The model under review builds one solid part; all positions refer to its coordinate system, in mm. A direction names the side the tool comes from. Give positions to 0.01 mm unless a question says otherwise; leave off trailing zeros. Order: outer loops, then holes, each group sorted by start corner. A loop starts at its lowest first (then second) coordinate and runs counter-clockwise, first axis right, second up.
Autodesk Inventor part; units mm, degrees
ref_plane "YZ Plane" through (0, 0, 0) normal (1, 0, 0) x (0, 1, 0)
ref_plane "XZ Plane" through (0, 0, 0) normal (0, 1, 0) x (-1, 0, 0)
ref_plane "XY Plane" through (0, 0, 0) normal (0, 0, 1) x (1, 0, 0)
sketch "Sketch1" plane through (0, 0, 0) normal (0, 1, 0) x (-1, 0, 0)
  point P0 (0, 0)
sketch "Sketch2" plane through (0, 0, 0) normal (0, 1, 0) x (-1, 0, 0)
  arc A0 (0, -12.775) -> (0, 12.775) centre (0, 0) ccw
  arc A1 (0, -27.775) -> (0, 27.775) centre (0, 0) ccw
  line L0 (0, 27.775) -> (0, -27.775)
  dimension "d0" = 25.55
  dimension "d1" = 15
extrude "Extrusion1" add sketch "Sketch2" along normal blind 14 contours A0 L0 A1
sketch "Sketch4" plane through (0, 0, 27.775) normal (1, 0, 0) x (0, 0, -1)
  line L0 (4.7364, 11.7377) -> (10.2211, 11.7622)
  line L1 (10.2211, 11.7622) -> (12.9848, 7.0245)
  line L2 (12.9848, 7.0245) -> (10.2636, 2.2623)
  line L3 (10.2636, 2.2623) -> (4.7789, 2.2378)
  line L4 (4.7789, 2.2378) -> (2.0152, 6.9755)
  line L5 (2.0152, 6.9755) -> (4.7364, 11.7377)
  line L6 (0, 14) -> (15, 14)
  line L7 (0, 0) -> (0, 14)
  line L8 (15, 14) -> (40.55, 14)
  line L9 (27.775, 14) -> (27.775, 0)
  line L10 (50.8136, 11.7377) -> (45.3289, 11.7622)
  line L11 (45.3289, 11.7622) -> (42.5652, 7.0245)
  line L12 (42.5652, 7.0245) -> (45.2864, 2.2623)
  line L13 (45.2864, 2.2623) -> (50.7711, 2.2378)
  line L14 (50.7711, 2.2378) -> (53.5348, 6.9755)
  line L15 (53.5348, 6.9755) -> (50.8136, 11.7377)
  line L16 (55.55, 14) -> (40.55, 14)
  line L17 (55.55, 0) -> (55.55, 14)
  line L18 (40.55, 14) -> (15, 14)
  point P0 (7.5, 7)
  point P1 (7.4787, 11.75)
  point P2 (7.5, 14)
  point P3 (0, 7)
  point P4 (48.05, 7)
  point P5 (48.0713, 11.75)
  point P6 (48.05, 14)
  point P7 (55.55, 7)
  dimension "d5" = 9.5
  dimension "d6" = 0
  dimension "d7" = 0
extrude "Extrusion2" cut sketch "Sketch4" against normal through all
sketch "Sketch5" plane through (0, 0, 27.775) normal (1, 0, 0) x (0, 0, -1)
  line L0 (4.7364, 11.7377) -> (10.2211, 11.7622)
  circle A0 centre (7.4787, 6.9999) radius 2.85
  line L1 (0.8522, 11.9261) -> (14.3606, 11.9261)
  line L2 (14.3606, 11.9261) -> (14.3606, 2.2036)
  line L3 (14.3606, 2.2036) -> (0.8522, 2.2036)
  line L4 (0.8522, 2.2036) -> (0.8522, 11.9261)
  line L5 (10.2636, 2.2623) -> (4.7789, 2.2378)
  line L6 (55.55, 14) -> (0, 14)
  line L7 (27.775, 14) -> (27.775, 0)
  line L8 (55.55, 0) -> (0, 0)
  line L9 (50.8136, 11.7377) -> (45.3289, 11.7622)
  circle A1 centre (48.0713, 6.9999) radius 2.85
  line L10 (54.6978, 11.9261) -> (41.1894, 11.9261)
  line L11 (41.1894, 11.9261) -> (41.1894, 2.2036)
  line L12 (41.1894, 2.2036) -> (54.6978, 2.2036)
  line L13 (54.6978, 2.2036) -> (54.6978, 11.9261)
  line L14 (45.2864, 2.2623) -> (50.7711, 2.2378)
  point P0 (7.4787, 11.75)
  point P1 (7.4787, 11.75)
  point P2 (48.0713, 11.75)
  point P3 (48.0713, 11.75)
  dimension "d12" = 5.7
  dimension "d13" = 0
  dimension "d14" = 4.75
extrude "Extrusion3" add sketch "Sketch5" against normal blind 6
sketch "Sketch6" plane through (-6, 0, 27.775) normal (-1, 0, 0) x (0, 0, 1)
  line L0 (-27.775, 0) -> (-27.775, 14)
  line L1 (-40.55, 14) -> (-15, 14)
  line L2 (-10.2636, 2.2623) -> (-4.7789, 2.2378)
  line L3 (-10.2636, 2.2623) -> (-4.7789, 2.2378)
  line L4 (-4.7789, 2.2378) -> (-2.0152, 6.9755)
  line L5 (-4.7789, 2.2378) -> (-2.0152, 6.9755)
  line L6 (-2.0152, 6.9755) -> (-4.7364, 11.7377)
  line L7 (-2.0152, 6.9755) -> (-4.7364, 11.7377)
  line L8 (-4.7364, 11.7377) -> (-10.2636, 11.7624)
  line L9 (-10.2636, 11.7624) -> (-13.0059, 7.0615)
  line L10 (-13.0059, 7.0615) -> (-10.2636, 2.2623)
  circle A0 centre (-7.4787, 6.9999) radius 2.85
  circle A1 centre (-7.4787, 6.9999) radius 7
  line L11 (-45.2864, 2.2623) -> (-50.7711, 2.2378)
  line L12 (-45.2864, 2.2623) -> (-50.7711, 2.2378)
  line L13 (-50.7711, 2.2378) -> (-53.5348, 6.9755)
  line L14 (-50.7711, 2.2378) -> (-53.5348, 6.9755)
  line L15 (-53.5348, 6.9755) -> (-50.8136, 11.7377)
  line L16 (-53.5348, 6.9755) -> (-50.8136, 11.7377)
  line L17 (-50.8136, 11.7377) -> (-45.2864, 11.7624)
  line L18 (-45.2864, 11.7624) -> (-42.5441, 7.0615)
  line L19 (-42.5441, 7.0615) -> (-45.2864, 2.2623)
  circle A2 centre (-48.0713, 6.9999) radius 2.85
  circle A3 centre (-48.0713, 6.9999) radius 7
  dimension "d17" = 14
extrude "Extrusion4" add sketch "Sketch6" along normal blind 12 and the other way blind 6 contours A1 | A3
properties part number "clamp_bolt"
Item 1: Take a section at D-D (x = -25.25). Give the boundary of the cut face in (y, z), and give its area (3 significant figures).
Values found:
outline: (0, -11.57) - (14, -11.57) - (14, 11.57) - (0, 11.57) - close
area: 324 mm2
Item 2: Take a section at C-C (x = -11.75). Give the boundary of the cut face in (y, z).
Values found:
outline: (0, -25.17) - (1.97, -25.17) arc R7 ccw to (12.03, -25.17) - (14, -25.17) - (14, -5.01) - (0, -5.01) - (0, -20.26) arc R7 ccw to (0, -20.33) - close; (0, 5.01) - (14, 5.01) - (14, 25.17) - (12.03, 25.17) arc R7 ccw to (1.97, 25.17) - (0, 25.17) - (0, 20.33) arc R7 ccw to (0, 20.26) - close; hole (2.24, -23) - (6.98, -25.76) - (11.74, -23.04) - (11.76, -17.55) - (7.02, -14.79) - (2.26, -17.51) - close; hole (2.24, 23) - (2.26, 17.51) - (7.02, 14.79) - (11.76, 17.55) - (11.74, 23.04) - (6.98, 25.76) - close
Item 3: For line 1 (Z direction, x = -6.25, y = 7.75); line 2 (Z direction, x = -8, y = 7); line 3 (Y direction, x = -15, z = 18), list the stretches that pass through material, from the lowest coordinate up.
Values found:
line 1: z = -27.26 to -25.32, -15.21 to -11.14, 11.14 to 15.21, 25.32 to 27.26
line 2: z = -27.3 to -25.75, -14.8 to -9.96, 9.96 to 14.8, 25.75 to 27.3
line 3: y = 0 to 2.26, 11.76 to 14
Item 4: Take a section at A-A (x = -2.25). Give the boundary of the cut face in (y, z).
Values found:
outline: (0, -27.68) - (14, -27.68) - (14, -12.58) - (0, -12.58) - (0, -20.26) arc R7 ccw to (0, -20.33) - close; (0, 12.58) - (14, 12.58) - (14, 27.68) - (0, 27.68) - (0, 20.33) arc R7 ccw to (0, 20.26) - close; hole circle Ø5.7 at (7, -20.3); hole circle Ø5.7 at (7, 20.3)
Item 5: Draft analysis for pull direction Y (two halves, no side actions). For faces 1 (the flat face through (-20.1, 4.68, -16.13)), 2 (the flat face through (0, 10, -20)), 3 (the flat face through (-14, 0, 0)), state which applies: released by +Y, released by -Y, zero draft, split by the parting line, or undercut.
Values found:
face 1: undercut
face 2: zero draft
face 3: released by -Y
Item 6: For faces 4 (the cylindrical face through (-12.907, 6.858, -27.295)), 5 (the flat face through (-18, 7, -26)), 6 (the flat face through (-11.916, 4.573, 24.359)), 7 (the cylindrical face through (-12.906, 7.142, 27.295)), list the 3-axis set-ups (+Z, -Z, +X, -X, +Y, -Y) from which the entire face can be reached by the end or side of a thin tool; tool diameter is ignored.
Values found:
face 4: -Z, -X
face 5: -Z, -X, +Y, -Y
face 6: -X
face 7: +Z, -X
Item 7: Take a section at B-B (z = 0). Give the boundary of the cut face in (x, y) (3 decimals).
Values found:
outline: (-27.775, 0) - (-12.775, 0) - (-12.775, 14) - (-27.775, 14) - close
Item 8: Clearance check with flat-ended pins moving along their axes: pin 1 Ø6 at (x, y) = (-9, 5.5) entering from -Z; pin 2 Ø7 at (y, z) = (9.5, 23.5) entering from -X; pin 3 Ø0.8 at (y, z) = (5.5, 16.5) entering from -X. State where each tip first meets the part, or that it passes through.
Values found:
pin 1: stops at z = -27.3
pin 2: stops at x = -18.39
pin 3: stops at x = -6
